```python
from build123d import *

# Parameters (mm, degrees)
SKETCH2_R               = 10
BOSS_EXTRUDE1_DEPTH     = 26.5
CUT_EXTRUDE1_DEPTH      = 44.029059948
CUT_EXTRUDE1_DEPTH_BACK = 44.029059948
SKETCH3_R               = 2.6
SKETCH12_R              = 14.5
CUT_EXTRUDE9_DEPTH      = 8.5
CHAMFER1_SIZE           = 0.6
FILLET1_R               = 0.39


with BuildPart() as part:
    # Sketch2 → Boss-Extrude1 (new, symmetric)
    with BuildSketch(Plane.XY):
        Polygon((-27, -20.5), (-13.931623932, -20.5), (-12.851623932, -19.42), (12.851623932, -19.42), (13.931623932, -20.5), (27, -20.5), (27, -10.58), (25.92, -9.5), (25.92, 14.5), (16.153846154, 14.5), (10, 20.5), (-10, 20.5), (-16.153846154, 14.5), (-25.92, 14.5), (-25.92, -9.5), (-27, -10.58), align=None)
        Circle(SKETCH2_R, mode=Mode.SUBTRACT)
    extrude(amount=BOSS_EXTRUDE1_DEPTH, both=True)

    # Sketch3 → Cut-Extrude1 (cut, two sides: drawn at the far end of the back side and taken through both)
    with BuildSketch(Plane(origin=(0, 0, 0), x_dir=(1, 0, 0), z_dir=(0, 1, 0)).offset(-CUT_EXTRUDE1_DEPTH_BACK)):
        with Locations((-20, 20)):
            Circle(SKETCH3_R)
        with Locations(Location((20, 20, 0), (0, 0, 90))):
            Circle(SKETCH3_R)
        with Locations(Location((20, -20, 0), (0, 0, 90))):
            Circle(SKETCH3_R)
        with Locations((-20, -20)):
            Circle(SKETCH3_R)
    extrude(amount=CUT_EXTRUDE1_DEPTH + CUT_EXTRUDE1_DEPTH_BACK, mode=Mode.SUBTRACT)

    # Sketch12 → Cut-Extrude9 (cut)
    with BuildSketch(Plane(origin=(0, 0, -26.5), x_dir=(-1, 0, 0), z_dir=(0, 0, -1))):
        Circle(SKETCH12_R)
    cut_extrude9 = extrude(amount=-CUT_EXTRUDE9_DEPTH, mode=Mode.SUBTRACT)

    # Mirror1: Cut-Extrude9 across plane
    add(cut_extrude9.mirror(Plane.XY), mode=Mode.SUBTRACT)

    # Chamfer1
    chamfer1_edges = [part.edges().sort_by_distance(p)[0] for p in [
        (-10, 0, -18),
        (14.5, 0, -26.5),
        (14.5, 0, 26.5),
        (-10, 0, 18),
    ]]
    chamfer(chamfer1_edges, length=CHAMFER1_SIZE)

    # Fillet1
    fillet1_edges = [part.edges().sort_by_distance(p)[0] for p in [
        (-27, -10.58, 0),
        (-25.92, -9.5, 0),
        (-25.92, 14.5, 0),
        (-16.153846154, 14.5, 0),
        (-10, 20.5, 0),
        (10, 20.5, 0),
        (16.153846154, 14.5, 0),
        (25.92, 14.5, 0),
        (25.92, -9.5, 0),
        (27, -10.58, 0),
        (27, -20.5, 0),
        (13.931623932, -20.5, 0),
        (12.851623932, -19.42, 0),
        (-12.851623932, -19.42, 0),
        (-13.931623932, -20.5, 0),
        (-27, -20.5, 0),
    ]]
    fillet(fillet1_edges, radius=FILLET1_R)


solid = part.part
```
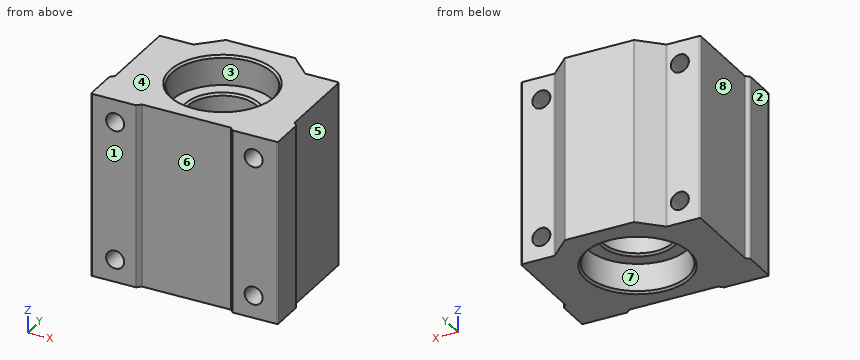
Build history of the part. All positions in model axes, mm. Face numbers are marked on the shaded views. A direction names the side the tool comes from. Round coordinates to 2 decimals unless told otherwise and drop trailing zeros. Write each loop counter-clockwise with the first axis right and the second up, starting at its lowest first coordinate (ties: lowest second). Pieces come first, ordered by that corner, then holes.
1) Drill centre lines: probe 1 along Z at (x, y) = (-20, 2.5); probe 2 along Z at (x, y) = (-19, 3.5); probe 3 along Y at (x, z) = (0, 4). Where is each one in solid material? Low to high.
2) Band-saw the part on B-B, the plane x = 0. List the corners of the cut face in (y, z).
3) Pin check, flat tips, straight feed: pin 1 (4.5 mm diameter, centred on x = 19, z = -12, fed in from +Y); pin 2 (8.5 mm diameter, centred on x = 0, y = 6.5, fed in from +Z); pin 3 (3 mm diameter, centred on x = 20, z = -20, fed in from +Y); pin 4 (7.5 mm diameter, centred on x = 2.5, z = -0.5, fed in from -Y). Stop position of each tip, or through.
4) Band-saw the part on D-D, the plane x = -20. List the corners of the cut face in (y, z).
5) 3-axis set-ups, long thin cutter, end or side, ignore diameter. For the marked faces 4, 5, 6, 7 and 8: which of +Z, -Z, +X, -X, +Y, -Y reach the whole face in a straight line?
6) Band-saw the part on A-A, the plane y = 0. List the corners of the cut face in (x, z), and give its area (3 significant figures).
7) Mould opens along X. For the marked faces 1, 2 and 3 say: +X half, -X half, draft (parallel to the pull), parting line (faces both ways), or undercut.
Ans:
1. probe 1: z = -26.5 to -22.6, -17.4 to 17.4, 22.6 to 26.5
1. probe 2: z = -26.5 to -22.4, -17.6 to 17.6, 22.4 to 26.5
1. probe 3: y = -19.42 to -10, 10 to 20.5
2. outline: (-19.42, -26.5) - (-15.1, -26.5) - (-14.5, -25.9) - (-14.5, -18) - (-10.6, -18) - (-10, -17.4) - (-10, 17.4) - (-10.6, 18) - (-14.5, 18) - (-14.5, 25.9) - (-15.1, 26.5) - (-19.42, 26.5) - close; (10, -17.4) - (10.6, -18) - (14.5, -18) - (14.5, -25.9) - (15.1, -26.5) - (20.5, -26.5) - (20.5, 26.5) - (15.1, 26.5) - (14.5, 25.9) - (14.5, 18) - (10.6, 18) - (10, 17.4) - close
3. pin 1: stops at y = 14.5
3. pin 2: stops at z = 18
3. pin 3: passes through
3. pin 4: stops at y = -19.42
4. outline: (-20.5, -26.5) - (14.5, -26.5) - (14.5, -22.6) - (-20.5, -22.6) - close; (-20.5, -17.4) - (14.5, -17.4) - (14.5, 17.4) - (-20.5, 17.4) - close; (-20.5, 22.6) - (14.5, 22.6) - (14.5, 26.5) - (-20.5, 26.5) - close
5. face 4: +Z, +X, -X, +Y, -Y
5. face 5: +Z, -Z, +X, +Y
5. face 6: +Z, -Z, -Y
5. face 7: -Z
5. face 8: +Z, -Z, -X, +Y
6. outline: (-25.92, -26.5) - (-15.1, -26.5) - (-14.5, -25.9) - (-14.5, -18) - (-10.6, -18) - (-10, -17.4) - (-10, 17.4) - (-10.6, 18) - (-14.5, 18) - (-14.5, 25.9) - (-15.1, 26.5) - (-25.92, 26.5) - close; (10, -17.4) - (10.6, -18) - (14.5, -18) - (14.5, -25.9) - (15.1, -26.5) - (25.92, -26.5) - (25.92, 26.5) - (15.1, 26.5) - (14.5, 25.9) - (14.5, 18) - (10.6, 18) - (10, 17.4) - close; hole circle Ø5.2 at (-20, -20); hole circle Ø5.2 at (-20, 20); hole circle Ø5.2 at (20, -20); hole circle Ø5.2 at (20, 20)
6. area: 1,450 mm2
7. face 1: draft
7. face 2: -X half
7. face 3: undercut
